Autodesk Fusion 360 part; units mm, degrees
sketch "Sketch1" plane through (0, 0, 0) normal (0, 0, 1) x (1, 0, 0)
  circle A0 centre (0, 0) radius 2.5
  circle A1 centre (0, 12) radius 2.5
  circle A2 centre (65, 0) radius 2.5
  circle A3 centre (0, 12) radius 5
  line L0 (5, -2) -> (60, -2)
  line L1 (5, 12) -> (5, -2)
  circle A4 centre (0, 0) radius 5
  line L2 (-5, 0) -> (-5, 12)
  line L3 (0, 0) -> (65, 0) construction
  line L4 (32.5, 0) -> (32.5, -19.0435) construction
  line L5 (4.5, -9.5218) -> (60.5, -9.5218) construction
  line L6 (-4.3911, -2.3912) -> (6.5, -22.3912)
  line L7 (6.5, -22.3912) -> (6.5, -67.3912)
  line L8 (6.5, -67.3912) -> (32.5, -67.3912)
  line L9 (58.5, -67.3912) -> (32.5, -67.3912)
  line L10 (58.5, -22.3912) -> (58.5, -67.3912)
  line L11 (69.3911, -2.3912) -> (58.5, -22.3912)
  circle A5 centre (65, 0) radius 5
  line L12 (70, 0) -> (70, 12)
  circle A6 centre (65, 12) radius 5
  line L13 (60, 12) -> (60, -2)
  circle A7 centre (65, 12) radius 2.5
  dimension "d1" = 5
  dimension "d2" = 5
  dimension "d3" = 5
  dimension "d5" = 12
  dimension "d6" = 65
  dimension "d9" = 2
  dimension "d10" = 10
  dimension "d12" = 56
  dimension "d13" = 45
  dimension "d14" = 26
  dimension "d15" = 20
extrude "Extrude1" add sketch "Sketch1" along normal blind 3.175
fillet "Fillet1" radius 5 6 edges at (5, -2, 1.5875) (60, -2, 1.5875) (58.5, -67.3912, 1.5875) (6.5, -67.3912, 1.5875) (58.5, -22.3912, 1.5875) (6.5, -22.3912, 1.5875)
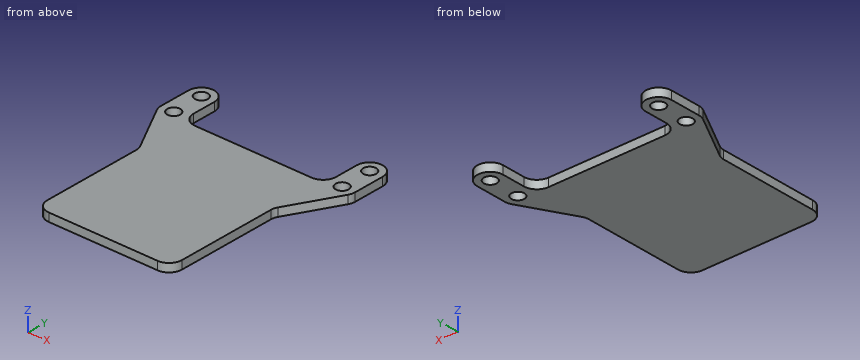
For this review, take the finished solid that the model builds, in its own axes (mm). Round coordinates to 2 decimals unless told otherwise and drop trailing zeros. Write each loop counter-clockwise with the first axis right and the second up, starting at its lowest first coordinate (ties: lowest second). Pieces come first, ordered by that corner, then holes. Notation, with made-up numbers: M 80.25,78 L 106.25,78 A18 ccw 106.25,107 Z; hole C -25.75,-21 d3. An arc over 180 degrees is marked long. Write item = value, one per line. Start each with the question number.
(1) For line 1 along Y through (x, z) = (65, 1.75); line 2 along Y through (x, z) = (-0.5, 1.25); line 3 along Y through (x, z) = (42, 2.2), list the stretches that pass through material, from the lowest coordinate up.
(2) We need section A-A (z = 2.5). Give the boundary of the cut face in (x, y).
(3) We need section D-D (x = 52.5). Give the boundary of the cut face in (y, z) (3 decimals).
(4) We need section C-C (y = -27.5). Give the boundary of the cut face in (x, z) (3 decimals), then the cut area to 3 significant figures.
(5) Clearance check with flat-ended pins moving along their axes: pin 1 Ø1.5 at (x, z) = (26.5, 1.5) entering from +Y; pin 2 Ø4 at (x, y) = (4, -47.5) entering from -Z; pin 3 Ø1.6 at (y, z) = (-51, 1.5) entering from -X; pin 4 Ø1 at (y, z) = (-38, 1.5) entering from +X. State where each tip first meets the part, or that it passes through.
(6) We need section B-B (x = 0). Give the boundary of the cut face in (y, z) (3 decimals), then the cut area to 3 significant figures.
Results found:
q1.line_1 = -10.45 to -2.5, 2.5 to 9.5, 14.5 to 17
q1.line_2 = -9.54 to -2.45, 2.45 to 9.55, 14.45 to 16.97
q1.line_3 = -67.39 to -2
q2.outline = M -5,0 A5 ccw -4.39,-2.39 L 5.89,-21.27 A5 cw 6.5,-23.66 L 6.5,-62.39 A5 ccw 11.5,-67.39 L 53.5,-67.39 A5 ccw 58.5,-62.39 L 58.5,-23.66 A5 cw 59.11,-21.27 L 69.39,-2.39 A5 ccw 70,0 L 70,12 A5 ccw 60,12 L 60,3 A5 cw 55,-2 L 10,-2 A5 cw 5,3 L 5,12 A5 ccw -5,12 Z; hole C 0,0 d5; hole C 0,12 d5; hole C 65,0 d5; hole C 65,12 d5
q3.outline = M -67.391,0 L -2,0 L -2,3.175 L -67.391,3.175 Z
q4.outline = M 6.5,0 L 58.5,0 L 58.5,3.175 L 6.5,3.175 Z
q4.area = 165 mm²
q5.pin_1 = -2
q5.pin_2 = through
q5.pin_3 = 6.5
q5.pin_4 = 58.5
q6.outline = M -10.455,0 L -2.5,0 L -2.5,3.175 L -10.455,3.175 Z; M 2.5,0 L 9.5,0 L 9.5,3.175 L 2.5,3.175 Z; M 14.5,0 L 17,0 L 17,3.175 L 14.5,3.175 Z
q6.area = 55.4 mm²
